For this review, take the finished solid that the model builds, in its own axes (mm). A direction names the side the tool comes from. Round coordinates to 2 decimals unless told otherwise and drop trailing zeros. Loops run counter-clockwise (first coordinate to the right, second up) from the corner with the lowest first, then second, coordinate; pieces in that order, holes last.
1) Tool access review of faces 4 (the flat face through (10, 2, -18)), 5 (the cylindrical face through (10.89, 23.69, -2.46)): name each direction out of +Z, -Z, +X, -X, +Y, -Y from which nothing blocks a thin tool from reaching the whole face with its end or side.
2) Take a section at D-D (z = -22.5). State the section outline as (x, y) points, then the cut area to 3 significant figures.
3) Wall thickness on L1, parallel to Y at x = 10, z = -2.85; L2, parallel to Z at x = 4.75, y = 19.5; L3, parallel to Y at x = 13.5, z = -9: over which ranges is each line inside the solid? List them lowest first.
4) Take a section at A-A (x = 10). State the section outline as (y, z) points, then the cut area to 3 significant figures.
5) Take a section at C-C (y = 22.3). State the section outline as (x, z) points.
6) Insertion check: pin 1 (6 mm diameter, centred on x = 12.5, z = -21, fed in from +Y); pin 2 (2.5 mm diameter, centred on x = 10, y = 22.3, fed in from -Z). Each pin has a flat end and moves straight along its axis. Give the tip position at first contact, or say it passes through.
7) Take a section at B-B (y = 8.25). State the section outline as (x, z) points.
8) Mouldability with a two-part tool opening along Y and no side actions: class faces 1 (the cylindrical face through (9.11, 23.69, -32.53)), 2 (the flat face through (17.963, 11.573, -32.535)), 3 (the flat face through (10, 12, 0)) as pulls with the +Y half, pulls with the -Y half, needs draft (parallel to the pull), parting line crosses it, or undercut.
```python
from build123d import *

# Parameters (mm, degrees)
SKETCH2_W                       = 20
SKETCH2_H                       = 35
BOSS_EXTRUDE2_DEPTH             = 2
BOSS_EXTRUDE5_DEPTH             = 5
BOSS_EXTRUDE6_DEPTH             = 5
FILLET1_R                       = 6
PREFORO_DA_MASCHIARE_M4_1_D     = 3.3
PREFORO_DA_MASCHIARE_M4_1_DEPTH = 5.000103078
PREFORO_DA_MASCHIARE_M4_2_D     = 3.3


with BuildPart() as part:
    # Sketch2 → Boss-Extrude2 (new body)
    with BuildSketch(Plane(origin=(0, 0, 0), x_dir=(1, 0, 0), z_dir=(0, 1, 0))):
        with Locations((10, 17.5)):
            Rectangle(SKETCH2_W, SKETCH2_H)
    extrude(amount=BOSS_EXTRUDE2_DEPTH)

    # 3DSketch3 → Boss-Extrude5 (add)
    with BuildSketch(Plane(origin=(10, 49, 0), x_dir=(-0.20810764446485872, -0.9781059289848355, 0), z_dir=(0, 0, 1))):
        Polygon((0, 0), (48.052055107, 0), (43.889902218, 19.56211858), align=None)
    extrude(amount=-BOSS_EXTRUDE5_DEPTH)

    # 3DSketch4 → Boss-Extrude6 (add)
    with BuildSketch(Plane(origin=(10, 2, -35), x_dir=(0, 1, 0), z_dir=(0, 0, 1))):
        Polygon((47, 0), (0, 10), (0, -10), align=None)
    extrude(amount=BOSS_EXTRUDE6_DEPTH)

    # Fillet1
    fillet1_edges = [part.edges().sort_by_distance(p)[0] for p in [
        (10, 49, -2.5),
        (10, 49, -32.5),
    ]]
    fillet(fillet1_edges, radius=FILLET1_R)

    # Preforo da maschiare M4-1
    with Locations(Plane.XY.offset(-30)):
        with Locations((10, 22.3)):
            Hole(PREFORO_DA_MASCHIARE_M4_1_D / 2, depth=PREFORO_DA_MASCHIARE_M4_1_DEPTH)

    # Preforo da maschiare M4-2 (through all)
    with Locations(Plane(origin=(0, 0, -5), x_dir=(-1, 0, 0), z_dir=(0, 0, -1))):
        with Locations((-10, 22.3)):
            Hole(PREFORO_DA_MASCHIARE_M4_2_D / 2)


solid = part.part
```
Response:
1. face 4: +X, -X, +Y
1. face 5: +Z, -Z
2. outline: (0, 0) - (20, 0) - (20, 2) - (0, 2) - close
2. area: 40.0 mm2
3. L1: y = 0 to 20.65, 23.95 to 26.17
3. L2: z = -35 to -30, -5 to 0
3. L3: y = 0 to 2
4. outline: (0, -35) - (20.65, -35) - (20.65, -30) - (2, -30) - (2, -5) - (20.65, -5) - (20.65, 0) - (0, 0) - close; (23.95, -35) - (26.17, -35) - (26.17, -30) - (23.95, -30) - close; (23.95, -5) - (26.17, -5) - (26.17, 0) - (23.95, 0) - close
4. area: 279 mm2
5. outline: (4.39, -35) - (8.35, -35) - (8.35, -30) - (4.39, -30) - close; (4.39, -5) - (8.35, -5) - (8.35, 0) - (4.39, 0) - close; (11.65, -35) - (15.61, -35) - (15.61, -30) - (11.65, -30) - close; (11.65, -5) - (15.61, -5) - (15.61, 0) - (11.65, 0) - close
6. pin 1: stops at y = 2
6. pin 2: passes through
7. outline: (1.33, -35) - (18.67, -35) - (18.67, -30) - (1.33, -30) - close; (1.33, -5) - (18.67, -5) - (18.67, 0) - (1.33, 0) - close
8. face 1: undercut
8. face 2: pulls with the +Y half
8. face 3: needs draft
